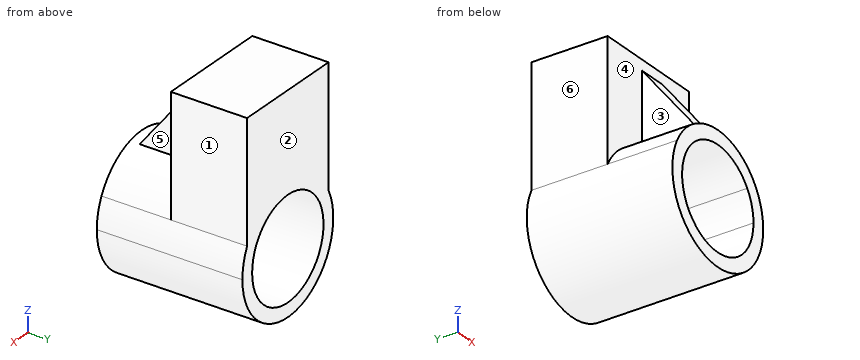
from build123d import *

# Parameters (mm, degrees)
F1_DEPTH = 25.4
F2_DEPTH = 48.514
F4_DEPTH = 19.304
F6_DEPTH = 25.4


with BuildPart() as f1:
    # F0 (on Front) → F1 (new body)
    with BuildSketch(Plane.XZ):
        with BuildLine():
            Line((-19.1385153821, 49.2832697928), (-19.1385153821, 9.4504378209))
            ThreePointArc((-19.1385153821, 9.4504378209), (0, 21.3446374071), (19.1385153821, 9.4504378209))
            Line((19.1385153821, 9.4504378209), (19.1590227187, 9.4504378209))
            Line((19.1590227187, 9.4504378209), (19.1590227187, 49.2832697928))
            Line((19.1590227187, 49.2832697928), (-19.1385153821, 49.2832697928))
        make_face()
    extrude(amount=F1_DEPTH)

    # F0 (on Front) → F2 (join)
    with BuildSketch(Plane.XZ):
        with BuildLine():
            ThreePointArc((19.1385153821, 9.4504378209), (0, 21.3446374071), (-19.1385153821, 9.4504378209))
            Line((-19.1385153821, 9.4504378209), (-13.8539659138, 9.4504378209))
            ThreePointArc((-13.8539659138, 9.4504378209), (0, 16.7703054995), (13.8539659138, 9.4504378209))
            Line((13.8539659138, 9.4504378209), (19.1385153821, 9.4504378209))
        make_face()
        with BuildLine():
            Line((-13.8539659138, 9.4504378209), (-19.1385153821, 9.4504378209))
            ThreePointArc((-19.1385153821, 9.4504378209), (-4.8522610553, -20.7857910287), (21.3446374071, 0))
            ThreePointArc((21.3446374071, 0), (20.7857910287, 4.8522610553), (19.1385153821, 9.4504378209))
            Line((19.1385153821, 9.4504378209), (13.8539659138, 9.4504378209))
            ThreePointArc((13.8539659138, 9.4504378209), (16.0246433237, 4.9450938208), (16.7703054995, 0))
            ThreePointArc((16.7703054995, 0), (-4.9450938208, -16.0246433237), (-13.8539659138, 9.4504378209))
        make_face()
    extrude(amount=F2_DEPTH)

    # F3 (on face) → F4 (join)
    with BuildSketch(Plane.XZ.offset(25.4)):
        with BuildLine():
            Line((-3.1239633907, 45.8474755287), (-3.1239633907, 21.1147909952))
            ThreePointArc((-3.1239633907, 21.1147909952), (0, 21.3446374071), (3.1239633907, 21.1147909952))
            Line((3.1239633907, 21.1147909952), (6.5980968066, 21.1147909952))
            Line((6.5980968066, 21.1147909952), (6.5980968066, 45.8474755287))
            Line((6.5980968066, 45.8474755287), (-3.1239633907, 45.8474755287))
        make_face()
    extrude(amount=F4_DEPTH)

    # F5 (on face) → F6 (cut)
    with BuildSketch(Plane.YZ.offset(6.5980968066)):
        Polygon((-44.704, 45.8474755287), (-44.704, 21.1147909952), (-25.4, 45.8474755287), align=None)
    extrude(amount=-F6_DEPTH, mode=Mode.SUBTRACT)


solid = f1.part
The model under review builds one solid part; all positions refer to its coordinate system, in mm. Face numbers are marked on the shaded views. A direction names the side the tool comes from. Give positions to 0.01 mm unless a question says otherwise; leave off trailing zeros. Write each loop counter-clockwise with the first axis right and the second up, starting at its lowest first coordinate (ties: lowest second). Pieces come first, ordered by that corner, then holes.
1. Tool access review of the marked faces 1, 2 and 3: name each direction out of +Z, -Z, +X, -X, +Y, -Y from which nothing blocks a thin tool from reaching the whole face with its end or side.
2. Add section D-D, the plane z = 40. Write out the cut boundary in (x, y), plus the area to 3 significant figures.
3. For P1, Ø12, axis at y = -27.5, z = 3, coming from the +X side; P2, Ø6, axis at x = 15.5, y = -35.5, coming from the -Z side; P3, Ø5, axis at x = 5.5, y = -30.5, coming from the +Z side; P4, Ø6, axis at x = -13.5, y = -18.5, coming from the -Z side, all flat-tipped, find the tip position at first contact; note any pin that passes through.
4. Wall thickness on L1, parallel to Z at x = 0, y = -22; L2, parallel to X at y = -15, z = 0; L3, parallel to Z at x = 5, y = -39: over which ranges is each line inside the solid? List them lowest first.
5. Add section A-A, the plane x = 0. Write out the cut boundary in (y, z), plus the area to 3 significant figures.
6. Draft analysis for pull direction X (two halves, no side actions). For the marked faces 4, 5 and 6, state which applies: +X half, -X half, draft (parallel to the pull), parting line (faces both ways), or undercut.
7. Add section C-C, the plane z = -1.5. Write out the cut boundary in (x, y).
Worked answers:
1. face 1: +Z, +X, +Y, -Y
1. face 2: +Z, -Z, +X, -X, +Y
1. face 3: +Z, -X, -Y
2. outline: (-19.14, -25.4) - (-3.12, -25.4) - (-3.12, -29.96) - (6.6, -29.96) - (6.6, -25.4) - (19.16, -25.4) - (19.16, 0) - (-19.14, 0) - close
2. area: 1,020 mm2
3. P1: stops at x = 21.34
3. P2: stops at z = -17.3
3. P3: stops at z = 42.52
3. P4: stops at z = -18.58
4. L1: z = -21.34 to -16.77, 16.77 to 49.28
4. L2: x = -21.34 to -16.77, 16.77 to 21.34
4. L3: z = -20.75 to -16.01, 16.01 to 20.75, 21.11 to 28.42
5. outline: (-48.51, -21.34) - (0, -21.34) - (0, -16.77) - (-48.51, -16.77) - close; (-48.51, 16.77) - (0, 16.77) - (0, 49.28) - (-25.4, 49.28) - (-25.4, 45.85) - (-44.7, 21.11) - (-44.7, 21.34) - (-48.51, 21.34) - close
5. area: 1,390 mm2
6. face 4: draft
6. face 5: +X half
6. face 6: -X half
7. outline: (-21.29, -48.51) - (-16.7, -48.51) - (-16.7, 0) - (-21.29, 0) - close; (16.7, -48.51) - (21.29, -48.51) - (21.29, 0) - (16.7, 0) - close
